Build history of the part. All positions in model axes, mm. A direction names the side the tool comes from. Round coordinates to 2 decimals unless told otherwise and drop trailing zeros. Write each loop counter-clockwise with the first axis right and the second up, starting at its lowest first coordinate (ties: lowest second). Pieces come first, ordered by that corner, then holes. Notation, with made-up numbers: (-37.5, 62) -> (-32.5, 62) arc R18 ccw to (-32.5, 96) -> close; hole circle Ø9 at (-7.75, 26.25). An arc over 180 degrees is marked (long way). Return JSON: item names as keys, results as strings.
from build123d import *

# Parameters (mm, degrees)
BOSS_EXTRUDE1_DEPTH         = 11.1125
SKETCH2_R                   = 3.5687
CUT_EXTRUDE1_DEPTH          = 38.600633721
SKETCH3_R                   = 3.5687
CUT_EXTRUDE2_DEPTH          = 38.600633721
F_3_8_16_TAPPED_HOLE1_D     = 7.9375
F_3_8_16_TAPPED_HOLE1_DEPTH = 23.8125
F_3_8_16_TAPPED_HOLE1_TIP   = 2.384665582


with BuildPart() as part:
    # Sketch1 → Boss-Extrude1 (new, symmetric)
    with BuildSketch(Plane.XY):
        with BuildLine():
            Line((0, 0), (0, 25.4))
            ThreePointArc((0, 25.4), (3.376576302, 24.001376302), (4.7752, 20.6248))
            Line((4.7752, 20.6248), (4.7752, 7.9502))
            ThreePointArc((4.7752, 7.9502), (5.70513597, 5.70513597), (7.9502, 4.7752))
            Line((7.9502, 4.7752), (20.6248, 4.7752))
            ThreePointArc((20.6248, 4.7752), (24.001376302, 3.376576302), (25.4, 0))
            Line((25.4, 0), (0, 0))
        make_face()
    extrude(amount=BOSS_EXTRUDE1_DEPTH, both=True)

    # Sketch2 → Cut-Extrude1 (cut, through all)
    with BuildSketch(Plane(origin=(0, 0, 0), x_dir=(1, 0, 0), z_dir=(0, 1, 0))):
        with Locations(Location((12.7, 0, 0), (0, 0, 90))):
            Circle(SKETCH2_R)
    extrude(amount=CUT_EXTRUDE1_DEPTH, mode=Mode.SUBTRACT)

    # Sketch3 → Cut-Extrude2 (cut, through all)
    with BuildSketch(Plane(origin=(0, 0, 0), x_dir=(0, 0, -1), z_dir=(1, 0, 0))):
        with Locations(Location((0, 12.7, 0), (0, 0, 270))):
            Circle(SKETCH3_R)
    extrude(amount=CUT_EXTRUDE2_DEPTH, mode=Mode.SUBTRACT)

    # 3/8-16 Tapped Hole1
    with Locations(Plane.ZY):
        with Locations((0, 12.7)):
            Hole(F_3_8_16_TAPPED_HOLE1_D / 2, depth=F_3_8_16_TAPPED_HOLE1_DEPTH)
            with Locations((0, 0, -(F_3_8_16_TAPPED_HOLE1_DEPTH + F_3_8_16_TAPPED_HOLE1_TIP / 2))):  # 118° drill point
                Cone(0, F_3_8_16_TAPPED_HOLE1_D / 2, F_3_8_16_TAPPED_HOLE1_TIP, mode=Mode.SUBTRACT)


solid = part.part
Q1. Saw through at B-B on x = 12.7. List the corners of the cut face in (y, z).
Verdict:
{"outline": "(0, -11.11) -> (4.78, -11.11) -> (4.78, -3.57) -> (0, -3.57) -> close; (0, 3.57) -> (4.78, 3.57) -> (4.78, 11.11) -> (0, 11.11) -> close"}
Q2. Two-plate mould, pull along X, no slides. Class faces 3 (the cylindrical face through (9.16, 2.35, 0.46)), 4 (the flat face through (16, 0, 3)), 5 (the cylindrical face through (5.68, 5.73, 0.16)): +X half, -X half, draft (parallel to the pull), parting line (faces both ways), or undercut.
Verdict:
{"face 3": "undercut", "face 4": "draft", "face 5": "+X half"}
Q3. Saw through at D-D on z = 7.5. List the corners of the cut face in (x, y) (3 decimals), then the cut area to 3 significant figures.
Verdict:
{"outline": "(0, 0) -> (25.4, 0) arc R4.775 ccw to (20.625, 4.775) -> (7.95, 4.775) arc R3.175 cw to (4.775, 7.95) -> (4.775, 20.625) arc R4.775 ccw to (0, 25.4) -> close", "area": "212 mm²"}
Q4. Saw through at A-A on y = 12.7. List the corners of the cut face in (x, z), then the cut area to 3 significant figures.
Verdict:
{"outline": "(0, -11.11) -> (4.78, -11.11) -> (4.78, -3.97) -> (0, -3.97) -> close; (0, 3.97) -> (4.78, 3.97) -> (4.78, 11.11) -> (0, 11.11) -> close", "area": "68.2 mm²"}
Q5. Pin check, flat tip, straight feed: pin 1 Ø9 at (y, z) = (12.7, 0) entering from +X. Stop position of the tip, or through.
Verdict:
{"pin 1": "stops at x = 4.78"}
Q6. 3-axis set-ups, long thin cutter, end or side, ignore diameter. For faces 1 (the flat face through (17, 4.775, 0)), 2 (the flat face through (7, 4, -11.112)): which of +Z, -Z, +X, -X, +Y, -Y reach the whole face in a straight line?
Verdict:
{"face 1": "+Z, -Z, +X, +Y", "face 2": "-Z, +X, -X, +Y, -Y"}
Q7. Wall check: L1, parallel to Z at x = 12.7, y = 1.45; L2, parallel to Y at x = 13.5, z = 5. Give the ranges that are in metal, low to high.
Verdict:
{"L1": "z = -11.11 to -3.57, 3.57 to 11.11", "L2": "y = 0 to 4.78"}
Q8. Saw through at C-C on z = 0. List the corners of the cut face in (x, y) (3 decimals), then the cut area to 3 significant figures.
Verdict:
{"outline": "(0, 0) -> (9.131, 0) -> (9.131, 4.775) -> (7.95, 4.775) arc R3.175 cw to (4.775, 7.95) -> (4.775, 8.731) -> (0, 8.731) -> close; (0, 16.669) -> (4.775, 16.669) -> (4.775, 20.625) arc R4.775 ccw to (0, 25.4) -> close; (16.269, 0) -> (25.4, 0) arc R4.775 ccw to (20.625, 4.775) -> (16.269, 4.775) -> close", "area": "140 mm²"}
